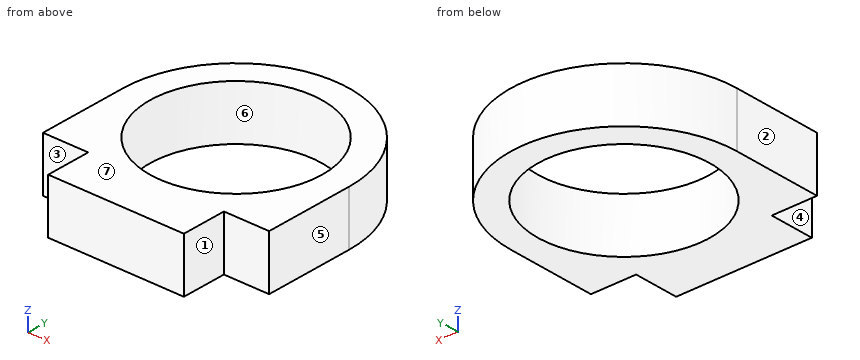
```python
from build123d import *

# Parameters (mm, degrees)
CROQUIS1_R              = 9.5
CROQUIS1_W              = 15
CROQUIS1_H              = 5
SALIENTE_EXTRUIR1_DEPTH = 6


with BuildPart() as part:
    # Croquis1 → Saliente-Extruir1 (new body)
    # profile 1 of 2: a face of its own
    with BuildSketch(Plane.XY):
        with BuildLine():
            Line((-12.5, 0), (-12.5, -10))
            Line((-12.5, -10), (-7.5, -10))
            Line((-7.5, -10), (7.5, -10))
            Line((7.5, -10), (12.5, -10))
            Line((12.5, -10), (12.5, 0))
            ThreePointArc((12.5, 0), (0, 12.5), (-12.5, 0))
        make_face()
        Circle(CROQUIS1_R, mode=Mode.SUBTRACT)
    # profile 2 of 2: a face of its own
    with BuildSketch(Plane.XY):
        with Locations((0, -12.5)):
            Rectangle(CROQUIS1_W, CROQUIS1_H)
    extrude(amount=SALIENTE_EXTRUIR1_DEPTH)


solid = part.part
```
Part model, mm, in its own coordinate system. Face numbers are marked on the shaded views. A direction names the side the tool comes from. Round coordinates to 2 decimals unless told otherwise and drop trailing zeros. Loops run counter-clockwise (first coordinate to the right, second up) from the corner with the lowest first, then second, coordinate; pieces in that order, holes last.
Item 1: Mould opens along X. For the marked faces 4, 5, 6 and 7 say: +X half, -X half, draft (parallel to the pull), parting line (faces both ways), or undercut.
Item 2: Cut at A-A, the plane x = 0. Give the cut face in (y, z), then the cut area to 3 significant figures.
Item 3: Drill centre lines: line 1 (Y direction, x = 0, z = 4.4); line 2 (X direction, y = 8.25, z = 4.5); line 3 (Y direction, x = 4.5, z = 1.5). Where is each one in solid material? Low to high.
Item 4: Drop flat-ended pins along their axis: P1, Ø2.5, axis at y = -12, z = 2, coming from the +X side; P2, Ø1.5, axis at x = 9, z = 2.5, coming from the -Y side; P3, Ø1.5, axis at y = -12, z = 1.5, coming from the -X side; P4, Ø8, axis at x = 4, y = 2.5, coming from the -Z side. Give the stop position or say it passes through.
Item 5: Cut at C-C, the plane z = 2.05. Give the cut face in (x, y), then the cut area to 3 significant figures.
Item 6: 3-axis set-ups, long thin cutter, end or side, ignore diameter. For the marked faces 1, 2 and 3: which of +Z, -Z, +X, -X, +Y, -Y reach the whole face in a straight line?
Item 7: Cut at B-B, the plane y = 3. Give the cut face in (x, z), then the cut area to 3 significant figures.
Item 8: Cut at D-D, the plane y = 11.25. Give the cut face in (x, z).
A:
1. face 4: -X half
1. face 5: +X half
1. face 6: undercut
1. face 7: draft
2. outline: (-15, 0) - (-9.5, 0) - (-9.5, 6) - (-15, 6) - close; (9.5, 0) - (12.5, 0) - (12.5, 6) - (9.5, 6) - close
2. area: 51.0 mm2
3. line 1: y = -15 to -9.5, 9.5 to 12.5
3. line 2: x = -9.39 to -4.71, 4.71 to 9.39
3. line 3: y = -15 to -8.37, 8.37 to 11.66
4. P1: stops at x = 7.5
4. P2: stops at y = -10
4. P3: stops at x = -7.5
4. P4: passes through
5. outline: (-12.5, -10) - (-7.5, -10) - (-7.5, -15) - (7.5, -15) - (7.5, -10) - (12.5, -10) - (12.5, 0) arc R12.5 ccw to (-12.5, 0) - close; hole circle Ø19 at (0, 0)
5. area: 287 mm2
6. face 1: +Z, -Z, +X, -Y
6. face 2: +Z, -Z, -X, +Y, -Y
6. face 3: +Z, -Z, -X, -Y
7. outline: (-12.13, 0) - (-9.01, 0) - (-9.01, 6) - (-12.13, 6) - close; (9.01, 0) - (12.13, 0) - (12.13, 6) - (9.01, 6) - close
7. area: 37.4 mm2
8. outline: (-5.45, 0) - (5.45, 0) - (5.45, 6) - (-5.45, 6) - close
